from build123d import *

# Parameters (mm, degrees)
F0_R     = 10
F1_DEPTH = 10
F2_R     = 4.25
F3_DEPTH = 10.001
F4_SIZE  = 5
F5_R     = 5


with BuildPart() as f1:
    # F0 (on Top) → F1 (new body)
    with BuildSketch(Plane.XY):
        Circle(F0_R)
    extrude(amount=F1_DEPTH)

    # F2 (on face) → F3 (cut, through all)
    with BuildSketch(Plane.XY.offset(10)):
        Circle(F2_R)
    extrude(amount=-F3_DEPTH, mode=Mode.SUBTRACT)

    # F4
    f4_edges = [f1.edges().sort_by_distance(p)[0] for p in [
        (-10, 0, 10),
    ]]
    chamfer(f4_edges, length=F4_SIZE)

    # F5
    f5_edges = [f1.edges().sort_by_distance(p)[0] for p in [
        (-10, 0, 5),
    ]]
    fillet(f5_edges, radius=F5_R)


solid = f1.part
Could you check a few things on this model? Use its own coordinates, in mm. Give positions to 0.01 mm unless a question says otherwise; leave off trailing zeros. Write each loop counter-clockwise with the first axis right and the second up, starting at its lowest first coordinate (ties: lowest second). Pieces come first, ordered by that corner, then holes. Notation, with made-up numbers: (58, 21) -> (101, 21) arc R23 ccw to (101, 37) -> close; hole circle Ø9 at (20.25, 38). An arc over 180 degrees is marked (long way). Answer as CSV lines item,"result". Start each with the question number.
(1) Please list where these lines run through material, in increasing order: line 1 (Y direction, x = 0, z = 3); line 2 (Y direction, x = 0, z = 5.5); line 3 (X direction, y = -2, z = 0.75).
(2) If we mould it in two halves opening along Y, with no side actions, what happens to faces 1 (the face through (-2, -4, 10)), 2 (the face through (-2.17, -9.76, 1.44)), 3 (the face through (2.285, 3.584, 5.07))? For each: +Y half, -Y half, draft (parallel to the pull), parting line (faces both ways), or undercut.
(3) I'm going to push flat-ended pins straight in: pin 1 Ø1.5 at (x, y) = (7.5, -1.5) entering from +Z; pin 2 Ø3 at (x, z) = (1.5, 9) entering from -Y; pin 3 Ø4 at (y, z) = (-4.5, 3) entering from -X; pin 4 Ø4 at (x, z) = (-2, 3) entering from +Y. Where does each tip first touch, or does it pass through?
(4) If we section it at A-A, the plane z = 8.5: Write out the boundary of the cut face in (x, y), and give its area (3 significant figures).
Answer list:
1,line 1,"-10 to -4.25, 4.25 to 10"
1,line 2,"-9.29 to -4.25, 4.25 to 9.29"
1,line 3,"-9.8 to -3.75, 3.75 to 9.8"
2,face 1,"draft"
2,face 2,"parting line"
2,face 3,"undercut"
3,pin 1,"z = 8.1"
3,pin 2,"y = -7.37"
3,pin 3,"x = -9.68"
3,pin 4,"y = 10"
4,outline,"circle Ø13 at (0, 0); hole circle Ø8.5 at (0, 0)"
4,area,"76.0 mm^2"
